Build history of the part. All positions in model axes, mm. Face numbers are marked on the shaded views. A direction names the side the tool comes from. Round coordinates to 2 decimals unless told otherwise and drop trailing zeros. Write each loop counter-clockwise with the first axis right and the second up, starting at its lowest first coordinate (ties: lowest second). Pieces come first, ordered by that corner, then holes. Notation, with made-up numbers: M 81,-5 L 89,-5 A5 ccw 89,-1 Z; hole C -26.5,45.25 d1. An arc over 180 degrees is marked long. Write item = value, one per line.
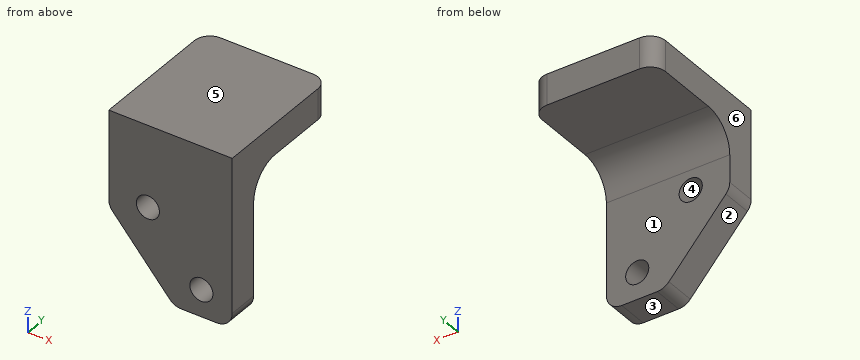
from build123d import *

# Parameters (mm, degrees)
BOSS_EXTRUDE1_DEPTH          = 4
SKETCH2_W                    = 16
SKETCH2_H                    = 18
BOSS_EXTRUDE2_DEPTH          = 4
FILLET1_R                    = 4
F_3_0_3_DIAMETER_HOLE1_D     = 3
F_3_0_3_DIAMETER_HOLE1_DEPTH = 30
F_3_0_3_DIAMETER_HOLE1_TIP   = 0.901290929
CUT_EXTRUDE1_DEPTH           = 10
FILLET2_R                    = 2


with BuildPart() as part:
    # Sketch1 → Boss-Extrude1 (new body)
    with BuildSketch(Plane.XY):
        with BuildLine():
            Line((0, 0), (0, 16))
            ThreePointArc((0, 16), (0.585786438, 17.414213562), (2, 18))
            Line((2, 18), (14, 18))
            ThreePointArc((14, 18), (15.414213562, 17.414213562), (16, 16))
            Line((16, 16), (16, 0))
            Line((16, 0), (0, 0))
        make_face()
    extrude(amount=BOSS_EXTRUDE1_DEPTH)

    # Sketch2 → Boss-Extrude2 (add)
    with BuildSketch(Plane(origin=(0, 0, 0), x_dir=(1, 0, 0), z_dir=(0, 1, 0))):
        with Locations((8, 9)):
            Rectangle(SKETCH2_W, SKETCH2_H)
    extrude(amount=BOSS_EXTRUDE2_DEPTH)

    # Fillet1
    fillet1_edges = [part.edges().sort_by_distance(p)[0] for p in [
        (8, 4, 0),
    ]]
    fillet(fillet1_edges, radius=FILLET1_R)

    # Ø3.0 (3) Diameter Hole1
    with Locations(Plane(origin=(939.624698197, 4, -711.338031018), x_dir=(-0.041819335, 0, -0.999125189), z_dir=(0, 1, 0))):
        with Locations((-665.06790374, 963.218082486), (-657.435781521, 955.954504856)):
            Hole(F_3_0_3_DIAMETER_HOLE1_D / 2, depth=F_3_0_3_DIAMETER_HOLE1_DEPTH)
            with Locations((0, 0, -(F_3_0_3_DIAMETER_HOLE1_DEPTH + F_3_0_3_DIAMETER_HOLE1_TIP / 2))):  # 118° drill point
                Cone(0, F_3_0_3_DIAMETER_HOLE1_D / 2, F_3_0_3_DIAMETER_HOLE1_TIP, mode=Mode.SUBTRACT)

    # Sketch6 → Cut-Extrude1 (cut)
    with BuildSketch(Plane(origin=(0, 4, 0), x_dir=(1, 0, 0), z_dir=(0, 1, 0))):
        Polygon((8.487460621, 18), (0, 8.300045005), (0, 18), align=None)
    extrude(amount=-CUT_EXTRUDE1_DEPTH, mode=Mode.SUBTRACT)

    # Fillet2
    fillet2_edges = [part.edges().sort_by_distance(p)[0] for p in [
        (16, 2, -18),
        (0, 2, -8.300045005),
        (8.487460621, 2, -18),
    ]]
    fillet(fillet2_edges, radius=FILLET2_R)


solid = part.part
1. Flat gauge pins, fed straight in: pin 1 (1 mm diameter, centred on x = 8.5, z = -4, fed in from +Y); pin 2 (4 mm diameter, centred on x = 5, y = 12.5, fed in from -Z). Where does each tip first touch, or does it go through?
Responses:
pin_1 = 4.03
pin_2 = 0
2. Mould opens along Z. For the marked faces 3, 4, 5 and 6 say: pulls with the +Z half, pulls with the -Z half, needs draft (parallel to the pull), parting line crosses it, or undercut.
Responses:
face_3 = pulls with the -Z half
face_4 = undercut
face_5 = pulls with the +Z half
face_6 = needs draft
3. Band-saw the part on C-C (y = 2). List the corners of the cut face in (x, z) (3 decimals), plus the area to 3 significant figures.
Responses:
outline = M 0,-7.549 A2 ccw 0.495,-8.866 L 7.89,-17.317 A2 ccw 9.395,-18 L 14,-18 A2 ccw 16,-16 L 16,4 L 0,4 Z; hole C 5.062,-6.571 d3; hole C 12,-14.5 d3
area = 296 mm²
4. Band-saw the part on A-A (x = 5.75). List the corners of the cut face in (y, z).
Responses:
outline = M 0,-14.87 L 4,-14.87 L 4,-7.9 L 0,-7.9 Z; M 0,-5.24 L 4,-5.24 L 4,-4 A4 cw 8,0 L 18,0 L 18,4 L 0,4 Z
5. Tool access for the marked faces 1 and 2: list every direction of +Z, -Z, +X, -X, +Y, -Y with a clear straight run to the whole face (end or side of a thin tool).
Responses:
face_1 = -Z, +X, -X, +Y
face_2 = -Z, -X, +Y, -Y
6. Probe probe 1 along Z at (x, y) = (12, 1.1); probe 2 along Z at (x, y) = (2.5, 14). List the from-to ranges inside material, lowest first.
Responses:
probe_1 = -18 to -16, -13 to 4
probe_2 = 0 to 4
7. Band-saw the part on D-D (x = 2.5). List the corners of the cut face in (y, z).
Responses:
outline = M 0,-11.16 L 4,-11.16 L 4,-4 A4 cw 8,0 L 18,0 L 18,4 L 0,4 Z
8. Band-saw the part on B-B (z = -14.5). List the corners of the cut face in (x, y).
Responses:
outline = M 5.42,0 L 10.5,0 L 10.5,4 L 5.42,4 Z; M 13.5,0 L 16,0 L 16,4 L 13.5,4 Z
